Design review of the part built by this model. Coordinates are the model's own, in mm. A direction names the side the tool comes from. Coordinates: 2 decimals unless noted, no trailing zeros. Write each loop counter-clockwise with the first axis right and the second up, starting at its lowest first coordinate (ties: lowest second). Pieces come first, ordered by that corner, then holes.
Q1. For probe 1 along Z at (x, y) = (7, -3); probe 2 along Z at (x, y) = (-3, 1.5); probe 3 along Z at (x, y) = (-14.5, 3.75), list the stretches that pass through material, from the lowest coordinate up.
Q2. Take a section at B-B (z = 7). Give the boundary of the cut face in (x, y), and give its area (3 significant figures).
Q3. Machinability: for faces 1 (the flat face through (-10, -2, -5)), 2 (the flat face through (-14.9, 9.9, -10)), 3 (the flat face through (-5, 10, -13)), which of the approach directions +Z, -Z, +X, -X, +Y, -Y give a long, thin tool a straight path to every point of the face, cutting with its end or side? Answer none if there is none.
Q4. Insertion check: pin 1 (7.5 mm diameter, centred on x = 4, y = 11, fed in from +Z); pin 2 (12 mm diameter, centred on y = 3, z = -16.5, fed in from +X); pin 3 (3 mm diameter, centred on y = 7, z = -10, fed in from -X); pin 4 (6 mm diameter, centred on x = 3.5, z = -4, fed in from +Y). Each pin has a flat end and moves straight along its axis. Give the tip position at first contact, or say it passes through.
Q5. Take a section at A-A (x = -7). Give the boundary of the cut face in (y, z), and give its area (3 significant figures).
Q6. Take a section at D-D (z = 0). Give the boundary of the cut face in (x, y), and give its area (3 significant figures).
Q7. Mouldability with a two-part tool opening along Y and no side actions: class faces 4 (the cylindrical face through (-25, 11, -15)), 5 (the flat face through (10, -2, -5)), 6 (the flat face through (2.395, 10.14, -17.535)) as pulls with the +Y half, pulls with the -Y half, needs draft (parallel to the pull), parting line crosses it, or undercut.
Q8. Take a section at C-C (x = -17). Give the boundary of the cut face in (y, z), and give its area (3 significant figures).
```python
from build123d import *

# Parameters (mm, degrees)
F0_R          = 1.75
F0_R_2        = 4
F0_W          = 5
F0_H          = 10
F1_DEPTH      = 5
F2_DEPTH      = 5
F2_DEPTH_BACK = 20
F3_R          = 5
F4_DEPTH      = 10
F6_DEPTH      = 5


with BuildPart() as f1:
    # F0 (on Front) → F1 (new body)
    with BuildSketch(Plane.XZ):
        Polygon((10, -10), (10, 10), (-10, 10), (-10, -10), (-5, -10), (-5, -20), (5, -20), (5, -10), align=None)
        with Locations((-7, -7)):
            Circle(F0_R, mode=Mode.SUBTRACT)
        with Locations((7, -7)):
            Circle(F0_R, mode=Mode.SUBTRACT)
        with Locations((-7, 7)):
            Circle(F0_R, mode=Mode.SUBTRACT)
        Circle(F0_R_2, mode=Mode.SUBTRACT)
        with Locations((7, 7)):
            Circle(F0_R, mode=Mode.SUBTRACT)
        with Locations((7.5, -15)):
            Rectangle(F0_W, F0_H)
    extrude(amount=F1_DEPTH)

    # F0 (on Front) → F2 (join, two sides)
    with BuildSketch(Plane.XZ) as f2_sk:
        with Locations((-7.5, -15)):
            Rectangle(F0_W, F0_H)
    extrude(amount=F2_DEPTH)
    extrude(f2_sk.sketch, amount=-F2_DEPTH_BACK)

    # F3 (on face) → F4 (join)
    with BuildSketch(Plane(origin=(0, 0, -20), x_dir=(1, 0, 0), z_dir=(0, 0, -1))):
        with BuildLine():
            Line((-21, -20), (-10, -20))
            Line((-10, -20), (-10, -2))
            Line((-10, -2), (-21, -2))
            ThreePointArc((-21, -2), (-27.3639610307, -4.6360389693), (-30, -11))
            ThreePointArc((-30, -11), (-27.3639610307, -17.3639610307), (-21, -20))
        make_face()
        with Locations((-20, -11)):
            Circle(F3_R, mode=Mode.SUBTRACT)
    extrude(amount=-F4_DEPTH)

    # F5 (on face) → F6 (join)
    with BuildSketch(Plane(origin=(0, 0, -20), x_dir=(1, 0, 0), z_dir=(0, 0, -1))):
        Polygon((-10, 5), (-10, 0), (-5, 0), (10, 0), (10, 5), align=None)
        Polygon((10, 0), (-5, 0), (-5, -20), align=None)
    extrude(amount=-F6_DEPTH)


solid = f1.part
```
Response:
1. probe 1: z = -20 to -8.75, -5.25 to 5.25, 8.75 to 10
1. probe 2: z = -20 to -15
1. probe 3: z = -20 to -10
2. outline: (-10, -5) - (-8.75, -5) - (-8.75, 0) - (-10, 0) - close; (-5.25, -5) - (5.25, -5) - (5.25, 0) - (-5.25, 0) - close; (8.75, -5) - (10, -5) - (10, 0) - (8.75, 0) - close
2. area: 65.0 mm2
3. face 1: +Z, -Z, -X, -Y
3. face 2: +Z, +X, -X, +Y
3. face 3: +Z, +X, +Y
4. pin 1: stops at z = -15
4. pin 2: stops at x = 10
4. pin 3: stops at x = -29.65
4. pin 4: stops at y = 0
5. outline: (-5, -20) - (20, -20) - (20, -10) - (0, -10) - (0, -8.75) - (-5, -8.75) - close; (-5, -5.25) - (0, -5.25) - (0, 5.25) - (-5, 5.25) - close; (-5, 8.75) - (0, 8.75) - (0, 10) - (-5, 10) - close
5. area: 315 mm2
6. outline: (-10, -5) - (-4, -5) - (-4, 0) - (-10, 0) - close; (4, -5) - (10, -5) - (10, 0) - (4, 0) - close
6. area: 60.0 mm2
7. face 4: undercut
7. face 5: needs draft
7. face 6: pulls with the +Y half
8. outline: (2, -20) - (7, -20) - (7, -10) - (2, -10) - close; (15, -20) - (20, -20) - (20, -10) - (15, -10) - close
8. area: 100 mm2
